The model under review builds one solid part; all positions refer to its coordinate system, in mm. A direction names the side the tool comes from. Coordinates: 2 decimals unless noted, no trailing zeros. Loops run counter-clockwise (first coordinate to the right, second up) from the corner with the lowest first, then second, coordinate; pieces in that order, holes last. Notation, with made-up numbers: (39.25, 56) -> (46.25, 56) arc R11 ccw to (46.25, 68) -> close; hole circle Ø4 at (80, 14). An arc over 180 degrees is marked (long way). One line per question, with ' | ' between items. Start each with the question number.
from build123d import *

# Parameters (mm, degrees)
BOSS_EXTRUDE1_DEPTH        = 155
FILLET1_R                  = 0.3
SKETCH2_R                  = 1.75
CUT_EXTRUDE1_DEPTH         = 155
SKETCH2_3_R                = 3
CUT_EXTRUDE2_DEPTH         = 3.5
CHAMFER1_SIZE              = 0.3
LPATTERN1_COUNT            = 8
LPATTERN1_PITCH            = 20
CHAMFER1_OF_LPATTERN1_SIZE = 0.3


with BuildPart() as part:
    # Sketch1 → Boss-Extrude1 (new body)
    with BuildSketch(Plane.XY):
        with BuildLine():
            Line((4.5, 2.75), (-4.5, 2.75))
            Line((-4.5, 2.75), (-4.5, 2.25))
            ThreePointArc((-4.5, 2.25), (-3.906959444, 2.05517259), (-3.545, 1.546605799))
            ThreePointArc((-3.545, 1.546605799), (-3.304423928, 1.477486263), (-3.2, 1.25))
            ThreePointArc((-3.2, 1.25), (-3.304423928, 1.022513737), (-3.545, 0.953394201))
            ThreePointArc((-3.545, 0.953394201), (-3.906959444, 0.44482741), (-4.5, 0.25))
            Line((-4.5, 0.25), (-4.5, -2.75))
            Line((-4.5, -2.75), (4.5, -2.75))
            Line((4.5, -2.75), (4.5, 0.25))
            ThreePointArc((4.5, 0.25), (3.906959444, 0.44482741), (3.545, 0.953394201))
            ThreePointArc((3.545, 0.953394201), (3.2, 1.25), (3.545, 1.546605799))
            ThreePointArc((3.545, 1.546605799), (3.906959444, 2.05517259), (4.5, 2.25))
            Line((4.5, 2.25), (4.5, 2.75))
        make_face()
    extrude(amount=BOSS_EXTRUDE1_DEPTH)

    # Fillet1
    fillet1_edges = [part.edges().sort_by_distance(p)[0] for p in [
        (-4.5, 2.75, 77.5),
        (4.5, 2.75, 77.5),
    ]]
    fillet(fillet1_edges, radius=FILLET1_R)

    # Sketch2 → Cut-Extrude1 (cut)
    with BuildSketch(Plane(origin=(0, 2.75, 0), x_dir=(1, 0, 0), z_dir=(0, 1, 0))):
        with Locations(Location((0, -7.5, 0), (0, 0, 180))):
            Circle(SKETCH2_R)
    cut_extrude1 = extrude(amount=-CUT_EXTRUDE1_DEPTH, mode=Mode.SUBTRACT)

    # Sketch2_3 → Cut-Extrude2 (cut)
    with BuildSketch(Plane(origin=(0, 2.75, 0), x_dir=(1, 0, 0), z_dir=(0, 1, 0))):
        with Locations(Location((0, -7.5, 0), (0, 0, 180))):
            Circle(SKETCH2_3_R)
    cut_extrude2 = extrude(amount=-CUT_EXTRUDE2_DEPTH, mode=Mode.SUBTRACT)

    # Chamfer1
    chamfer1_edges = [part.edges().sort_by_distance(p)[0] for p in [
        (1.75, -0.75, 7.5),
        (3, 2.75, 7.5),
    ]]
    chamfer(chamfer1_edges, length=CHAMFER1_SIZE)

    # LPattern1: Cut-Extrude1, Cut-Extrude2 ×8
    with Locations(*[(0, 0, i * LPATTERN1_PITCH) for i in range(1, LPATTERN1_COUNT)]):
        add(cut_extrude1, mode=Mode.SUBTRACT)
        add(cut_extrude2, mode=Mode.SUBTRACT)

    # Chamfer1 of LPattern1
    chamfer1_of_lpattern1_edges = [part.edges().sort_by_distance(p)[0] for p in [
        (1.75, -0.75, 27.5),
        (3, 2.75, 27.5),
        (1.75, -0.75, 47.5),
        (3, 2.75, 47.5),
        (1.75, -0.75, 67.5),
        (3, 2.75, 67.5),
        (1.75, -0.75, 87.5),
        (3, 2.75, 87.5),
        (1.75, -0.75, 107.5),
        (3, 2.75, 107.5),
        (1.75, -0.75, 127.5),
        (3, 2.75, 127.5),
        (1.75, -0.75, 147.5),
        (3, 2.75, 147.5),
    ]]
    chamfer(chamfer1_of_lpattern1_edges, length=CHAMFER1_OF_LPATTERN1_SIZE)


solid = part.part
1) Wall thickness on L1, parallel to Y at x = 3.5, z = 41; L2, parallel to Y at x = 4.25, z = 46; L3, parallel to X at y = 1.25, z = 39: over which ranges is each line inside the solid? List them lowest first.
2) Consider section A-A, the plane z = 107.5. Write out the cut boundary in (x, y) (3 decimals), plus the area to 3 significant figures.
3) Machinability: for faces 1 (the face through (0.65, 0.87, 64.57)), 2 (the face through (-0.9, -1.9, 149)), which of the approach directions +Z, -Z, +X, -X, +Y, -Y give a long, thin tool a straight path to every point of the face, cutting with its end or side? Answer none if there is none.
4) Insertion check: pin 1 Ø3 at (y, z) = (2, 32) entering from -X; pin 2 Ø4.5 at (x, z) = (0, 47.5) entering from +Y. Each pin has a flat end and moves straight along its axis. Give the tip position at first contact, or say it passes through.
5) Consider section B-B, the plane x = 0. Give the number of separate pieces and of enclosed holes in the cut face, plus the area to 3 significant figures.
6) Mouldability with a two-part tool opening along Z and no side actions: class faces 3 (the face through (-4.5, -1, 76)), 4 (the face through (-1.61, 0.87, 130.03)), 5 (the face through (0, 0, 155)) as +Z half, -Z half, draft (parallel to the pull), parting line (faces both ways), or undercut.
Filled sheet:
1) L1: -2.75 to 0.95, 1.55 to 2.75 | L2: -2.75 to 0.28, 2.22 to 2.75 | L3: -3.2 to 3.2
2) outline: (-4.5, -2.75) -> (-1.75, -2.75) -> (-1.75, -1.05) -> (-2.05, -0.75) -> (-3, -0.75) -> (-3, 2.45) -> (-3.3, 2.75) -> (-4.2, 2.75) arc R0.3 ccw to (-4.5, 2.45) -> (-4.5, 2.25) arc R1 cw to (-3.545, 1.547) arc R0.3 cw (long way) to (-3.545, 0.953) arc R1 cw to (-4.5, 0.25) -> close; (1.75, -2.75) -> (4.5, -2.75) -> (4.5, 0.25) arc R1 cw to (3.545, 0.953) arc R0.3 cw (long way) to (3.545, 1.547) arc R1 cw to (4.5, 2.25) -> (4.5, 2.45) arc R0.3 ccw to (4.2, 2.75) -> (3.3, 2.75) -> (3, 2.45) -> (3, -0.75) -> (2.05, -0.75) -> (1.75, -1.05) -> close | area: 17.8 mm^2
3) face 1: +Y | face 2: +Y, -Y
4) pin 1: x = -4.5 | pin 2: y = -0.75
5) separate pieces: 9 | enclosed holes: 0 | area: 627 mm^2
6) face 3: draft | face 4: undercut | face 5: +Z half
